Part model, mm, in its own coordinate system. A direction names the side the tool comes from. Give positions to 0.01 mm unless a question says otherwise; leave off trailing zeros. Order: outer loops, then holes, each group sorted by start corner. A loop starts at its lowest first (then second) coordinate and runs counter-clockwise, first axis right, second up. Notation, with made-up numbers: M 37,66.5 L 70,66.5 A17 cw 70,94.5 Z; hole C -8.75,74.5 d11. An arc over 180 degrees is marked long. Answer as a JSON object with one key per item and string values.
Autodesk Inventor part; units mm, degrees
ref_plane "YZ Plane" through (0, 0, 0) normal (1, 0, 0) x (0, 1, 0)
ref_plane "XZ Plane" through (0, 0, 0) normal (0, 1, 0) x (-1, 0, 0)
ref_plane "XY Plane" through (0, 0, 0) normal (0, 0, 1) x (1, 0, 0)
sketch "Sketch1" plane through (0, 0, 0) normal (0, 1, 0) x (-1, 0, 0)
  circle A0 centre (0, 0) radius 3.175
  circle A1 centre (0, 0) radius 1.9558
  dimension "d0" = 6.35
  dimension "d1" = 3.9116
extrude "Extrusion1" add sketch "Sketch1" along normal blind 6.35 contours A0 | A1
extrude "Extrusion2" add sketch "Sketch1" against normal blind 9.525 contours A1
fillet "Fillet1" radius 0.3175 4 edges at (3.175, 6.35, 0) (1.9558, -9.525, 0) (3.175, 0, 0) (1.9558, 0, 0)
properties part number "locatingpin" material "Silver"
1. Cut at D-D on y = -5. Give the cut face in (x, z).
Worked answers:
{"outline": "C 0,0 d3.91"}
2. Probe line 1 along Y through (x, z) = (0.25, -2.5); line 2 along Y through (x, z) = (2, 0.25); line 3 along X through (y, z) = (-2.25, 0.75). List the from-to ranges inside material, lowest first.
Worked answers:
{"line 1": "y = 0 to 6.35", "line 2": "y = -0.13 to 6.35", "line 3": "x = -1.81 to 1.81"}
3. Pin check, flat tips, straight feed: P1, Ø2, axis at x = -2, y = 0, coming from the -Z side; P2, Ø1.5, axis at y = -5.5, z = 0, coming from the -X side; P3, Ø1, axis at x = 2, y = -1, coming from the -Z side; P4, Ø1.5, axis at x = -1.5, z = -2.5, coming from the +Y side. Stop position of each tip, or through.
Worked answers:
{"P1": "stops at z = -3", "P2": "stops at x = -1.96", "P3": "stops at z = -1.26", "P4": "stops at y = 6.35"}
4. Which spindle directions (+Z, -Z, +X, -X, +Y, -Y) get a long thin tool onto all of the face, cutting with end or side? Do faces 1 (the flat face through (0, 6.35, 0)), 2 (the cylindrical face through (-1.865, -4.7, 0.587)). Say none if no direction does.
Worked answers:
{"face 1": "+Z, -Z, +X, -X, +Y", "face 2": "-Y"}
5. Cut at C-C on y = 3. Give the cut face in (x, z) (3 decimals), plus the area to 3 significant figures.
Worked answers:
{"outline": "C 0,0 d6.35", "area": "31.7 mm^2"}
